from build123d import *

# Parameters (mm, degrees)
ESBO_O1_W                = 182
ESBO_O1_H                = 131
ESBO_O1_W_2              = 171.2
ESBO_O1_H_2              = 112.2
RESSALTO_EXTRUS_O1_DEPTH = 2.5
ESBO_O1_4_W              = 171.2
ESBO_O1_4_H              = 112.2
ESBO_O1_4_W_2            = 160
ESBO_O1_4_H_2            = 96
RESSALTO_EXTRUS_O2_DEPTH = 0.5
ESBO_O2_W                = 32
ESBO_O2_H                = 30.698097853
CORTE_EXTRUS_O1_DEPTH    = 221.523241406


with BuildPart() as part:
    # Esboço1 → Ressalto-extrusão1 (new body)
    with BuildSketch(Plane.XY):
        with Locations((91, 65.5)):
            Rectangle(ESBO_O1_W, ESBO_O1_H)
        with Locations((91, 62.6)):
            Rectangle(ESBO_O1_W_2, ESBO_O1_H_2, mode=Mode.SUBTRACT)
    extrude(amount=RESSALTO_EXTRUS_O1_DEPTH)

    # Esboço1<4> → Ressalto-extrusão2 (add)
    with BuildSketch(Plane.XY):
        with Locations((91, 62.6)):
            Rectangle(ESBO_O1_4_W, ESBO_O1_4_H)
        with Locations((91, 65.5)):
            Rectangle(ESBO_O1_4_W_2, ESBO_O1_4_H_2, mode=Mode.SUBTRACT)
    extrude(amount=RESSALTO_EXTRUS_O2_DEPTH)

    # Esboço2 → Corte-extrusão1 (cut, through all)
    with BuildSketch(Plane(origin=(0, 6.5, 0), x_dir=(1, 0, 0), z_dir=(0, 1, 0))):
        with Locations((91, -15.849048927)):
            Rectangle(ESBO_O2_W, ESBO_O2_H)
    extrude(amount=-CORTE_EXTRUS_O1_DEPTH, mode=Mode.SUBTRACT)


solid = part.part
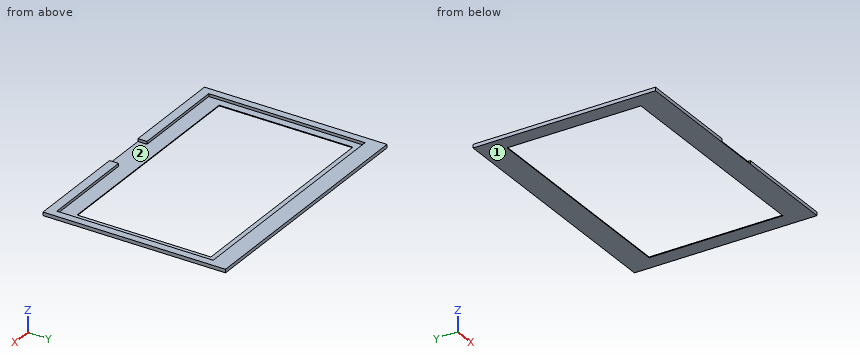
Build history of the part. All positions in model axes, mm. Face numbers are marked on the shaded views. Round coordinates to 2 decimals unless told otherwise and drop trailing zeros. Write each loop counter-clockwise with the first axis right and the second up, starting at its lowest first coordinate (ties: lowest second). Pieces come first, ordered by that corner, then holes. Notation, with made-up numbers: (-15.75, 15) -> (11.25, 15) arc R15 ccw to (11.25, 43) -> close; hole circle Ø10 at (46, 20.25). An arc over 180 degrees is marked (long way). Use one line per item in the form item = value.
Q1. Band-saw the part on B-B, the plane y = 68. Write the cut outline in (x, z), then the cut area to 3 significant figures.
Conclusion:
outline = (0, 0) -> (11, 0) -> (11, 0.5) -> (5.4, 0.5) -> (5.4, 2.5) -> (0, 2.5) -> close; (171, 0) -> (182, 0) -> (182, 2.5) -> (176.6, 2.5) -> (176.6, 0.5) -> (171, 0.5) -> close
area = 32.6 mm²
Q2. Band-saw the part on D-D, the plane y = 115.5. Write the cut outline in (x, z).
Conclusion:
outline = (0, 0) -> (182, 0) -> (182, 2.5) -> (176.6, 2.5) -> (176.6, 0.5) -> (5.4, 0.5) -> (5.4, 2.5) -> (0, 2.5) -> close
Q3. Band-saw the part on A-A, the plane x = 84. Write the cut outline in (y, z), then the cut area to 3 significant figures.
Conclusion:
outline = (0, 0) -> (17.5, 0) -> (17.5, 0.5) -> (0, 0.5) -> close; (113.5, 0) -> (131, 0) -> (131, 2.5) -> (118.7, 2.5) -> (118.7, 0.5) -> (113.5, 0.5) -> close
area = 42.1 mm²
Q4. Drill centre lines: L1, parallel to Y at x = 152.5, z = 0.3; L2, parallel to Y at x = 166.5, z = 1.9; L3, parallel to X at y = 29.5, z = 1.45. Where is each one in solid material? Low to high.
Conclusion:
L1 = 0 to 17.5, 113.5 to 131
L2 = 0 to 6.5, 118.7 to 131
L3 = 0 to 5.4, 176.6 to 182
Q5. Drop a flat-ended pin along its axis: P1, Ø0.6, axis at x = 54.5, z = 2, coming from the -Y side. Give the stop position or say it passes through.
Conclusion:
P1 = 0
Q6. Two-plate mould, pull along Y, no slides. Class the marked faces 1 and 2: released by +Y, released by -Y, zero draft, split by the parting line, or undercut.
Conclusion:
face_1 = zero draft
face_2 = undercut
Q7. Band-saw the part on C-C, the plane z = 1.9. Write the cut outline in (x, y).
Conclusion:
outline = (0, 0) -> (75, 0) -> (75, 6.5) -> (5.4, 6.5) -> (5.4, 118.7) -> (176.6, 118.7) -> (176.6, 6.5) -> (107, 6.5) -> (107, 0) -> (182, 0) -> (182, 131) -> (0, 131) -> close
